Geometry: see drawing. Coordinates: mm, zero at the bounding-box minimum. A direction names the side the tool comes from. Round coordinates to 2 decimals unless told otherwise and drop trailing zeros. Loops run counter-clockwise (first coordinate to the right, second up) from the corner with the lowest first, then second, coordinate; pieces in that order, holes last. Notation, with made-up numbers: (4.5, 78.5) - (16.5, 78.5) arc R17 ccw to (16.5, 84.5) - close; hole circle Ø4 at (89, 52.5). An arc over 180 degrees is marked (long way). Write item = value, one per line. Start each with the question number.
Item 1: Section A-A (y = 11.75). Return loops of the section in (x, z).
Item 2: Section B-B (x = 8.5). Return loops of the section in (y, z).
Item 3: First-contact query: pin 1 (1.4 mm diameter, centred on y = 9, z = 3.5, fed in from -X); pin 2 (2.5 mm diameter, centred on x = 11, z = 3.5, fed in from -Y); pin 3 (2.5 mm diameter, centred on y = 9.5, z = 3.5, fed in from +X); pin 4 (2 mm diameter, centred on x = 3.5, z = 3, fed in from -Y). Flat tips, straight axial feed; report the tip coordinate or a pass-through.
Item 4: Section C-C (z = 4.15). Return loops of the section in (x, y), plus the area to 3 significant figures.
Item 5: Line query: line 1 (Z direction, x = 4, y = 13); line 2 (X direction, y = 5.75, z = 3.15); line 3 (Y direction, x = 8, z = 2.5). Output: solid intervals per line, ascending. Write a range as from..to.
Item 6: Section D-D (x = 4.5). Return loops of the section in (y, z).
Item 7: Access query for the marked faces 1, 2 and 3. Directions: +Z, -Z, +X, -X, +Y, -Y. A direction counts if a zero-diameter tool reaches every point of the face in a straight line with its end or side. Return the directions, or none.
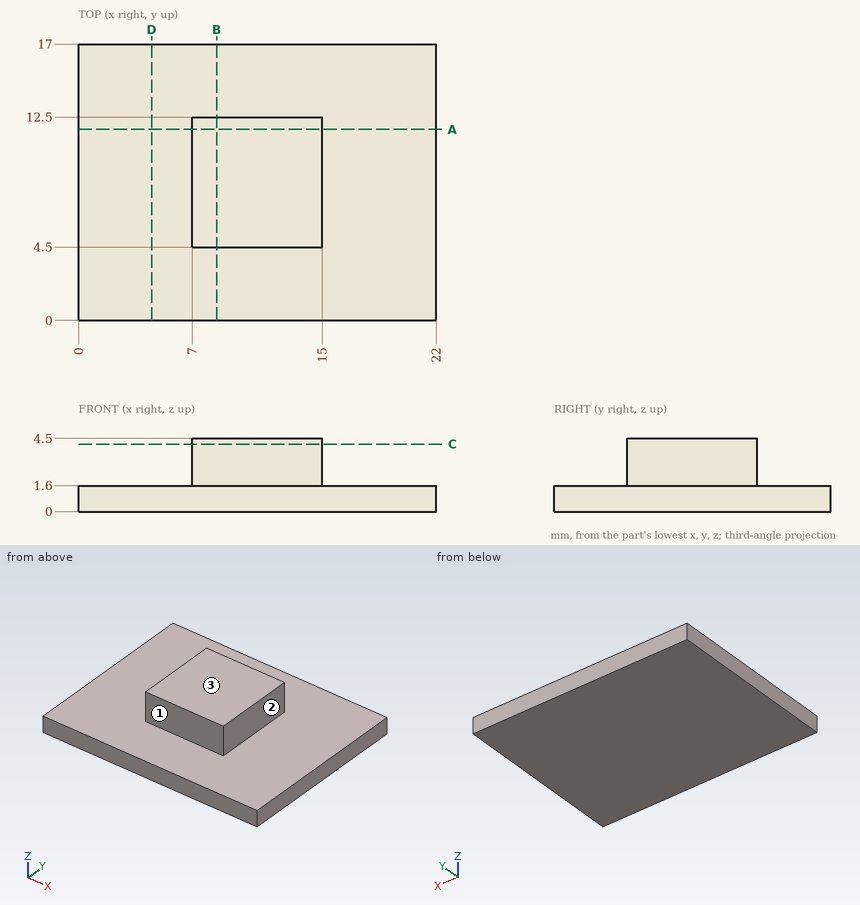
Taken from the geometry:
q1.outline = (0, 0) - (22, 0) - (22, 1.6) - (15, 1.6) - (15, 4.5) - (7, 4.5) - (7, 1.6) - (0, 1.6) - close
q2.outline = (0, 0) - (17, 0) - (17, 1.6) - (12.5, 1.6) - (12.5, 4.5) - (4.5, 4.5) - (4.5, 1.6) - (0, 1.6) - close
q3.pin_1 = 7
q3.pin_2 = 4.5
q3.pin_3 = 15
q3.pin_4 = through
q4.outline = (7, 4.5) - (15, 4.5) - (15, 12.5) - (7, 12.5) - close
q4.area = 64.0 mm^2
q5.line_1 = 0..1.6
q5.line_2 = 7..15
q5.line_3 = 4.5..12.5
q6.outline = (0, 0) - (17, 0) - (17, 1.6) - (0, 1.6) - close
q7.face_1 = +Z, +X, -X, -Y
q7.face_2 = +Z, +X, +Y, -Y
q7.face_3 = +Z, +X, -X, +Y, -Y
